from build123d import *

# Parameters (mm, degrees)
SKETCH1_W                = 55
SKETCH1_H                = 5
BOSS_EXTRUDE1_DEPTH      = 6
SKETCH1_4_R              = 6.5
BOSS_EXTRUDE2_DEPTH      = 3.5
BOSS_EXTRUDE3_DEPTH      = 10.5
BOSS_EXTRUDE3_DEPTH_BACK = 3.5
SKETCH1_5_R              = 6.5
SKETCH1_5_R_2            = 4
CUT_EXTRUDE1_REACH       = 44.03
SKETCH2_R                = 2.4


with BuildPart() as part:
    # Sketch1 → Boss-Extrude1 (new, symmetric)
    with BuildSketch(Plane.XY):
        Rectangle(SKETCH1_W, SKETCH1_H)
    extrude(amount=BOSS_EXTRUDE1_DEPTH, both=True)

    # Sketch1_4 → Boss-Extrude2 (add, symmetric)
    # profile 1 of 3: a face of its own
    with BuildSketch(Plane.XY):
        with BuildLine():
            Line((-14, 13.5), (-14, 2.5))
            Line((-14, 2.5), (-8.660254038, 2.5))
            ThreePointArc((-8.660254038, 2.5), (-12.594513816, 7.386226882), (-14, 13.5))
        make_face()
    # profile 2 of 3: a face of its own
    with BuildSketch(Plane.XY):
        with BuildLine():
            ThreePointArc((-14, 13.5), (-12.594513816, 7.386226882), (-8.660254038, 2.5))
            Line((-8.660254038, 2.5), (8.660254038, 2.5))
            ThreePointArc((8.660254038, 2.5), (12.594513816, 7.386226882), (14, 13.5))
            ThreePointArc((14, 13.5), (0, 27.5), (-14, 13.5))
        make_face()
        with Locations((0, 13.5)):
            Circle(SKETCH1_4_R, mode=Mode.SUBTRACT)
    # profile 3 of 3: a face of its own
    with BuildSketch(Plane.XY):
        with BuildLine():
            ThreePointArc((14, 13.5), (12.594513816, 7.386226882), (8.660254038, 2.5))
            Line((8.660254038, 2.5), (14, 2.5))
            Line((14, 2.5), (14, 13.5))
        make_face()
    extrude(amount=BOSS_EXTRUDE2_DEPTH, both=True)

    # Sketch1_5 → Boss-Extrude3 (add, two sides: drawn at the far end of the back side and taken through both)
    with BuildSketch(Plane.XY.offset(-BOSS_EXTRUDE3_DEPTH_BACK)):
        with Locations((0, 13.5)):
            Circle(SKETCH1_5_R)
        with Locations((0, 13.5)):
            Circle(SKETCH1_5_R_2, mode=Mode.SUBTRACT)
    extrude(amount=BOSS_EXTRUDE3_DEPTH + BOSS_EXTRUDE3_DEPTH_BACK)

    # Sketch2 → Cut-Extrude1 (cut, up to next)
    with BuildSketch(Plane.XZ.offset(2.5), mode=Mode.PRIVATE) as cut_extrude1_sk1:
        with Locations(Location((21, 0, 0), (0, 0, 270))):
            Circle(SKETCH2_R)
    cut_extrude1_tool1 = extrude(cut_extrude1_sk1.sketch, amount=-CUT_EXTRUDE1_REACH, mode=Mode.PRIVATE) & part.part
    # Sketch2 → Cut-Extrude1 (cut, up to next)
    with BuildSketch(Plane.XZ.offset(2.5), mode=Mode.PRIVATE) as cut_extrude1_sk2:
        with Locations(Location((-21, 0, 0), (0, 0, 270))):
            Circle(SKETCH2_R)
    cut_extrude1_tool2 = extrude(cut_extrude1_sk2.sketch, amount=-CUT_EXTRUDE1_REACH, mode=Mode.PRIVATE) & part.part
    add(cut_extrude1_tool1.solids().sort_by_distance((21, -2.5, 0))[0], mode=Mode.SUBTRACT)
    add(cut_extrude1_tool2.solids().sort_by_distance((-21, -2.5, 0))[0], mode=Mode.SUBTRACT)


solid = part.part
Work out the finished part from the listing and answer in its coordinate system (mm). A direction names the side the tool comes from. Give positions to 0.01 mm unless a question says otherwise; leave off trailing zeros. Loops run counter-clockwise (first coordinate to the right, second up) from the corner with the lowest first, then second, coordinate; pieces in that order, holes last. Notation, with made-up numbers: M 11.5,51 L 46.5,51 A22 ccw 46.5,86 Z; hole C 42.5,71.25 d9. An arc over 180 degrees is marked long. Use CSV: the item, a comma, the result in double quotes.
1) Find section A-A on z = 0. Write down the section's boundary in (x, y).
Answer:
outline,"M -27.5,-2.5 L -23.4,-2.5 L -23.4,2.5 L -27.5,2.5 Z; M -18.6,-2.5 L 18.6,-2.5 L 18.6,2.5 L 14,2.5 L 14,13.5 A14 ccw -14,13.5 L -14,2.5 L -18.6,2.5 Z; M 23.4,-2.5 L 27.5,-2.5 L 27.5,2.5 L 23.4,2.5 Z; hole C 0,13.5 d8"
2) Consider L1, parallel to X at y = 0.75, z = 0; L2, parallel to Y at x = 0, z = -0.25; L3, parallel to Y at x = 0, z = 6.75. Determine where each line is inside the solid, lowest interval first.
Answer:
L1,"-27.5 to -23.4, -18.6 to 18.6, 23.4 to 27.5"
L2,"-2.5 to 9.5, 17.5 to 27.5"
L3,"7 to 9.5, 17.5 to 20"
3) Find section B-B on x = 0. Write down the section's boundary in (y, z).
Answer:
outline,"M -2.5,-6 L 2.5,-6 L 2.5,-3.5 L 9.5,-3.5 L 9.5,10.5 L 7,10.5 L 7,3.5 L 2.5,3.5 L 2.5,6 L -2.5,6 Z; M 17.5,-3.5 L 27.5,-3.5 L 27.5,3.5 L 20,3.5 L 20,10.5 L 17.5,10.5 Z"
4) Find section C-C on z = 5. Write down the section's boundary in (x, y), plus the area to 3 significant figures.
Answer:
outline,"M -27.5,-2.5 L 27.5,-2.5 L 27.5,2.5 L -27.5,2.5 Z; C 0,13.5 d13; hole C 0,13.5 d8"
area,"357 mm^2"
5) Given P1, Ø6, axis at x = 21, z = 0, coming from the +Y side; P2, Ø3, axis at y = 6.5, z = 2, coming from the -X side; P3, Ø3, axis at x = -14, y = 15.5, coming from the -Z side, each flat-ended and moving along its own axis, determine where each tip first touches the part or whether it passes through.
Answer:
P1,"y = 2.5"
P2,"x = -14"
P3,"z = -3.5"
6) Determine the mould class of faces 1 (the cylindrical face through (-23.343, -0.035, 0.52)), 2 (the cylindrical face through (0.308, 27.497, 0.049)), 3 (the cylindrical face through (-0.521, 17.466, 3.402)), 4 (the flat face through (0, -2.5, 0)) for opening direction Y: released by +Y, released by -Y, zero draft, split by the parting line, or undercut.
Answer:
face 1,"zero draft"
face 2,"released by +Y"
face 3,"undercut"
face 4,"released by -Y"
7) Which of the six approach directions +Z, -Z, +X, -X, +Y, -Y give full straight-line access (tool end or side, diameter ignored) to faces 5 (the flat face through (-14, 8, 0)), 6 (the cylindrical face through (-0.846, 19.945, 6.951)), 7 (the flat face through (0, 18, -3.5)), 8 (the flat face through (14, 8, 0))?
Answer:
face 5,"+Z, -Z, -X, +Y"
face 6,"+Z"
face 7,"-Z, +X, -X, +Y"
face 8,"+Z, -Z, +X, +Y"
8) Find section D-D on y = 11. Write down the section's boundary in (x, z).
Answer:
outline,"M -14,-3.5 L -3.12,-3.5 L -3.12,10.5 L -6,10.5 L -6,3.5 L -14,3.5 Z; M 3.12,-3.5 L 14,-3.5 L 14,3.5 L 6,3.5 L 6,10.5 L 3.12,10.5 Z"
